Source: CAD feature listing. Evaluate the final solid. Frame: model axes, mm. Round coordinates to 2 decimals unless told otherwise and drop trailing zeros. Loops run counter-clockwise (first coordinate to the right, second up) from the corner with the lowest first, then second, coordinate; pieces in that order, holes last. Notation, with made-up numbers: (31.5, 37) -> (85.5, 37) arc R13 ccw to (85.5, 62) -> close; hole circle Ø3 at (13.25, -5.75). An arc over 180 degrees is marked (long way). Put each result on its own line as item: value. Start each with the question number.
1. Cut plane A-A (x = 54). Return the cut outline in (y, z).
2. Material intervals for L1, parallel to X at y = 2.95, z = -43.5; L2, parallel to X at y = 3.65, z = -57.5; L3, parallel to X at y = 2.6, z = -10.5, sorted ascending.
3. Contact query for flat-ended pins moving along their axis: pin 1 (1.2 mm diameter, centred on y = 2.5, z = -8, fed in from -X); pin 2 (1.2 mm diameter, centred on x = 212, y = 2.5, fed in from +Z); pin 3 (12 mm diameter, centred on x = 113, z = -14, fed in from -Y); pin 4 (1.2 mm diameter, centred on y = 2.5, z = -69, fed in from +X). Output: stop coordinate, or through.
4. Cut plane B-B (y = 3.05). State how many separate pieces and enclosed holes the cut face has, then the cut area to 3 significant figures.
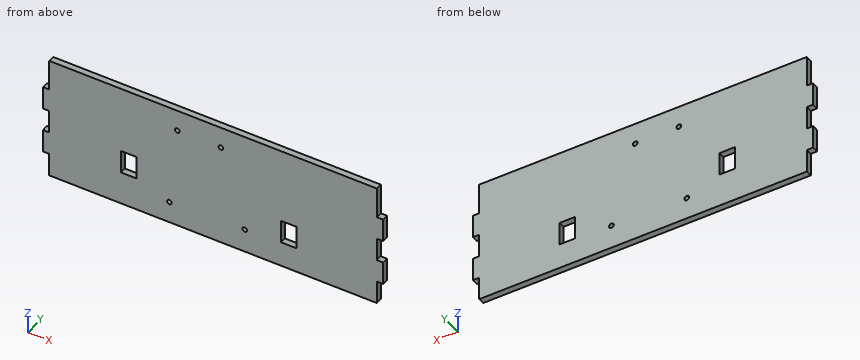
```python
from build123d import *

# Parameters (mm, degrees)
SKETCH1_W                       = 210
SKETCH1_H                       = 80
BOSS_EXTRUDE1_DEPTH             = 4
SKETCH2_W                       = 10
SKETCH2_H                       = 15
CUT_EXTRUDE1_DEPTH              = 225.757647256
SKETCH3_W                       = 15
SKETCH3_H                       = 4
BOSS_EXTRUDE2_DEPTH             = 4
SKETCH4_W                       = 15
SKETCH4_H                       = 4
BOSS_EXTRUDE3_DEPTH             = 4
F_3_0MM_DOWEL_HOLE1_D           = 3
F_3_0MM_DOWEL_HOLE1_CSINK_D     = 3.05
F_3_0MM_DOWEL_HOLE1_CSINK_ANGLE = 90


with BuildPart() as part:
    # Sketch1 → Boss-Extrude1 (new body)
    with BuildSketch(Plane(origin=(0, 0, 0), x_dir=(1, 0, 0), z_dir=(0, 1, 0))):
        with Locations((105, 40)):
            Rectangle(SKETCH1_W, SKETCH1_H)
    extrude(amount=BOSS_EXTRUDE1_DEPTH)

    # Sketch2 → Cut-Extrude1 (cut, through all)
    with BuildSketch(Plane(origin=(0, 4, 0), x_dir=(1, 0, 0), z_dir=(0, 1, 0))):
        with Locations((153.509116539, 56.141774946)):
            Rectangle(SKETCH2_W, SKETCH2_H)
        with Locations((51.014837185, 50.904860517)):
            Rectangle(SKETCH2_W, SKETCH2_H)
    extrude(amount=-CUT_EXTRUDE1_DEPTH, mode=Mode.SUBTRACT)

    # Sketch3 → Boss-Extrude2 (add)
    with BuildSketch(Plane.ZY):
        with Locations((-57.5, 2)):
            Rectangle(SKETCH3_W, SKETCH3_H)
        with Locations((-27.5, 2)):
            Rectangle(SKETCH3_W, SKETCH3_H)
    extrude(amount=BOSS_EXTRUDE2_DEPTH)

    # Sketch4 → Boss-Extrude3 (add)
    with BuildSketch(Plane(origin=(210, 0, 0), x_dir=(0, 0, -1), z_dir=(1, 0, 0))):
        with Locations((57.5, 2)):
            Rectangle(SKETCH4_W, SKETCH4_H)
        with Locations((27.5, 2)):
            Rectangle(SKETCH4_W, SKETCH4_H)
    extrude(amount=BOSS_EXTRUDE3_DEPTH)

    # Ø3.0mm Dowel Hole1 (through all)
    with Locations(Plane(origin=(0, 4, 0), x_dir=(1, 0, 0), z_dir=(0, 1, 0))):
        with Locations((125.265241585, 64.631998291), (77.005241585, 65.901998291), (82.085241585, 13.831998291), (110.025241585, 13.831998291)):
            CounterSinkHole(F_3_0MM_DOWEL_HOLE1_D / 2, F_3_0MM_DOWEL_HOLE1_CSINK_D / 2, counter_sink_angle=F_3_0MM_DOWEL_HOLE1_CSINK_ANGLE)


solid = part.part
```
Solution:
1. outline: (0, -80) -> (4, -80) -> (4, -58.4) -> (0, -58.4) -> close; (0, -43.4) -> (4, -43.4) -> (4, 0) -> (0, 0) -> close
2. L1: x = 0 to 46.01, 56.01 to 210
2. L2: x = -4 to 46.01, 56.01 to 148.51, 158.51 to 214
2. L3: x = 0 to 210
3. pin 1: stops at x = 0
3. pin 2: stops at z = -20
3. pin 3: stops at y = 0
3. pin 4: stops at x = 210
4. separate pieces: 1
4. enclosed holes: 6
4. area: 16,700 mm^2
